from build123d import *

# Parameters (mm, degrees)
F0_R           = 7.9375
F0_R_2         = 6.6548
F0_R_3         = 1.5875
F1_DEPTH       = 25.4
F3_D           = 7.9375
F3_DEPTH       = 19.05
F3_CSINK_D     = 9.525
F3_CSINK_ANGLE = 60
F3_TIP         = 2.3846655818
F4_DEPTH       = 0.381
F5_R           = 7.0485
F5_R_2         = 1.5875
F6_DEPTH       = 2.667
F7_SIZE        = 0.254


with BuildPart() as f1:
    # F0 (on Front) → F1 (new body)
    with BuildSketch(Plane.XZ):
        Circle(F0_R)
        Circle(F0_R_2, mode=Mode.SUBTRACT)
        Circle(F0_R_2)
        Circle(F0_R_3, mode=Mode.SUBTRACT)
    extrude(amount=-F1_DEPTH)

    # F3
    with Locations(Plane(origin=(0, 25.4, 0), x_dir=(-1, 0, 0), z_dir=(0, 1, 0))):
        with Locations((0, 0)):
            CounterSinkHole(F3_D / 2, F3_CSINK_D / 2, depth=F3_DEPTH, counter_sink_angle=F3_CSINK_ANGLE)
            with Locations((0, 0, -(F3_DEPTH + F3_TIP / 2))):  # 118° drill point
                Cone(0, F3_D / 2, F3_TIP, mode=Mode.SUBTRACT)

    # F0 (on Front) → F4 (join)
    with BuildSketch(Plane.XZ):
        Circle(F0_R_2)
        Circle(F0_R_3, mode=Mode.SUBTRACT)
    extrude(amount=F4_DEPTH)

    # F5 (on face) → F6 (join)
    with BuildSketch(Plane.XZ.offset(0.381)):
        Circle(F5_R)
        Circle(F5_R_2, mode=Mode.SUBTRACT)
    extrude(amount=F6_DEPTH)

    # F7
    f7_edges = [f1.edges().sort_by_distance(p)[0] for p in [
        (-7.0485, -3.048, 0),
        (-7.0485, -0.381, 0),
    ]]
    chamfer(f7_edges, length=F7_SIZE)


solid = f1.part
Geometry: final body of the model. Coordinates: model frame, mm. A direction names the side the tool comes from. Give positions to 0.01 mm unless a question says otherwise; leave off trailing zeros. Loops run counter-clockwise (first coordinate to the right, second up) from the corner with the lowest first, then second, coordinate; pieces in that order, holes last. Notation, with made-up numbers: (-34.5, -2) - (13.5, -2) arc R31 cw to (13.5, 33) - close; hole circle Ø2 at (2.5, -31). An arc over 180 degrees is marked (long way). Answer as CSV lines item,"result". Start each with the question number.
1. Section C-C, the plane y = 12.25. Return loops of the section in (x, z) (1 decimal), plus the area to 3 significant figures.
2. Draft query along Y for faces 1 (the face through (-5.593, -1.699, -4.289)), 2 (the face through (-1.66, 5.01, 0.52)), 3 (the face through (-7, 0, 2)). Return one class per face: released by +Y, released by -Y, zero draft, split by the parting line, or undercut.
3. Reachability of faces 4 (the face through (-0.86, 15.064, -3.874)), 5 (the face through (0, 25.4, -5)), 6 (the face through (-1.443, -0.188, -6.497)) from +Z, -Z, +X, -X, +Y, -Y: full face, straight path, thin tool, end or side. Return the list, or none.
4. Ray query, L1, parallel to Z at x = 0, y = -2.3; L2, parallel to Z at x = 0, y = 11; L3, parallel to X at y = 5.25, z = -1. Return the intervals inside material, ascending.
5. Pin query (flat end, axial travel): P1, Ø1, axis at x = -1.5, y = 1.5, coming from the +Z side; P2, Ø3, axis at x = -4.5, y = 0.5, coming from the -Z side; P3, Ø1.5, axis at x = 4.5, y = 1.5, coming from the +Z side. Return the tip coordinate at first contact, or that it passes through.
Answers:
1,outline,"circle Ø15.9 at (0, 0); hole circle Ø7.9 at (0, 0)"
1,area,"148 mm2"
2,face 1,"zero draft"
2,face 2,"released by +Y"
2,face 3,"undercut"
3,face 4,"+Y"
3,face 5,"+Z, -Z, +X, -X, +Y"
3,face 6,"none"
4,L1,"z = -7.05 to -1.59, 1.59 to 7.05"
4,L2,"z = -7.94 to -3.97, 3.97 to 7.94"
4,L3,"x = -7.87 to -1.89, 1.89 to 7.87"
5,P1,"stops at z = 7.87"
5,P2,"stops at z = -7.35"
5,P3,"stops at z = 7"
